Here's how the part is built. I have some questions about the finished solid (model axes, mm). Give positions to 0.01 mm unless a question says otherwise; leave off trailing zeros. Order: outer loops, then holes, each group sorted by start corner. A loop starts at its lowest first (then second) coordinate and runs counter-clockwise, first axis right, second up. Notation, with made-up numbers: (77.5, 80.5) -> (88.5, 80.5) arc R23 cw to (88.5, 106.5) -> close; hole circle Ø5 at (21.5, 47.25). An arc over 180 degrees is marked (long way). Write each question's results on one line, items separated by ' | '. Start each with the question number.
Q1. I'm going to push flat-ended pins straight in: pin 1 (1 mm diameter, centred on x = -4, z = 4.5, fed in from -Y); pin 2 (1.5 mm diameter, centred on y = -3, z = 3, fed in from -X). Where does each tip first touch, or does it pass through?
Q2. Thinking about a two-plate mould opening in X: for faces 1 (the face through (-3, 0, 2)), 2 (the face through (0, -4.72, 2)), 3 (the face through (4.07, -2.39, 2.47)), which applies, pulls with the +X half, pulls with the -X half, needs draft (parallel to the pull), parting line crosses it, or undercut?
Q3. I need wall thicknesses on line 1 along Y through (x, z) = (-1.25, 0.75); line 2 along Y through (x, z) = (0, 2); line 3 along X through (y, z) = (-2, 1.7). Which ranges of each line are inside material? Lowest first, please. Write a range as [from, to].
Q4. Imagine slicing it at B-B, the plane z = 3.75. Please give me the cut outline in (x, y) (3 decimals).
```python
from build123d import *

# Parameters (mm, degrees)
SKETCH1_R           = 3
BOSS_EXTRUDE1_DEPTH = 5
CHAMFER1_SIZE       = 0.25


with BuildPart() as part:
    # Sketch1 → Boss-Extrude1 (new body)
    with BuildSketch(Plane.XY):
        Polygon((5.45, 0), (2.725, 4.719838451), (-2.725, 4.719838451), (-5.45, 0), (-2.725, -4.719838451), (2.725, -4.719838451), align=None)
        Circle(SKETCH1_R, mode=Mode.SUBTRACT)
    extrude(amount=BOSS_EXTRUDE1_DEPTH)

    # Chamfer1
    chamfer1_edges = [part.edges().sort_by_distance(p)[0] for p in [
        (-3, 0, 0),
        (-3, 0, 5),
    ]]
    chamfer(chamfer1_edges, length=CHAMFER1_SIZE)

    # Sketch2 → Cut-Revolve1 (revolve, cut)
    with BuildSketch(Plane(origin=(0, 0, 0), x_dir=(1, 0, 0), z_dir=(0, 1, 0)), mode=Mode.PRIVATE) as cut_revolve1_sk:
        Polygon((-1, -5.5), (-4, -5.5), (-6.14222201, -4), (-6.14222201, -1), (-4, 0.5), (-1, 0.5), (-1, 1.980198167), (-7.750900281, 1.980198167), (-7.750900281, -6.98400312), (-1, -6.98400312), align=None)
    revolve(cut_revolve1_sk.sketch.rotate(Axis((0, 0, 5.5), (0, 0, -1)), 180), axis=Axis((0, 0, 5.5), (0, 0, -1)), mode=Mode.SUBTRACT)


solid = part.part
```
Geometry check:
1) pin 1: y = -3.38 | pin 2: x = -4.15
2) face 1: undercut | face 2: needs draft | face 3: pulls with the +X half
3) line 1: [-4.72, -2.73], [2.73, 4.72] | line 2: [-4.72, -3], [3, 4.72] | line 3: [-4.3, -2.24], [2.24, 4.3]
4) outline: (-5.45, 0) -> (-2.725, -4.72) -> (2.725, -4.72) -> (5.45, 0) -> (2.725, 4.72) -> (-2.725, 4.72) -> close; hole circle Ø6 at (0, 0)
